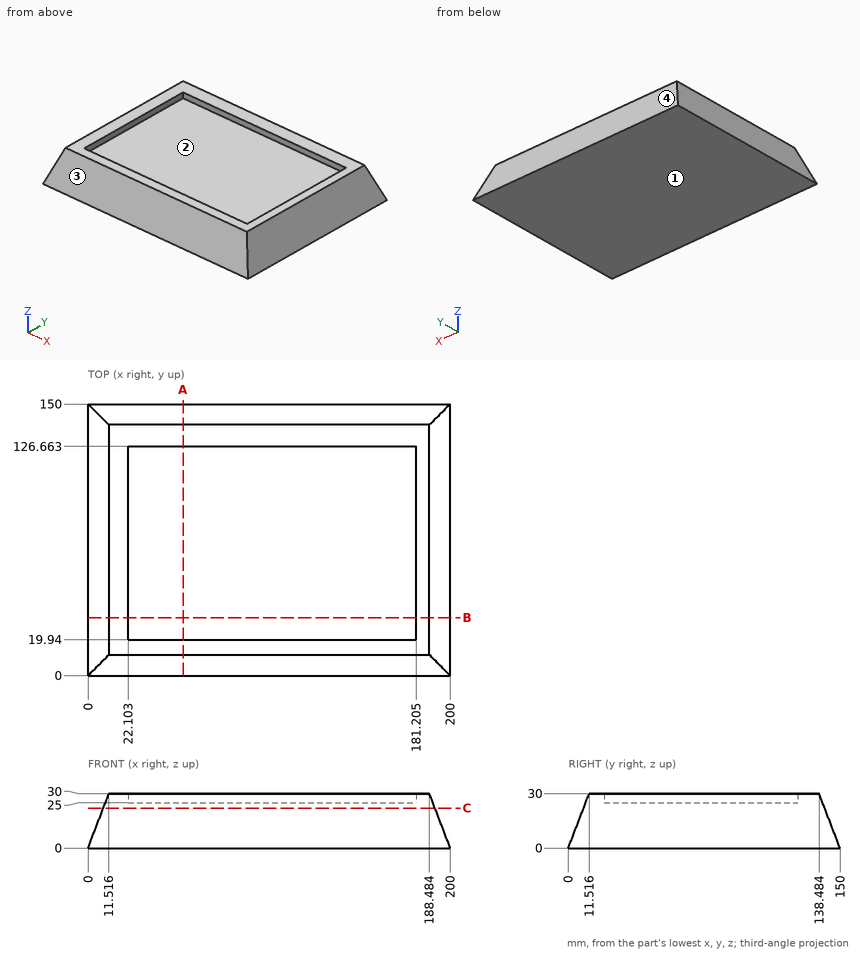
Could you check a few things on this drawing? It's one solid part, dimensions in mm from its lowest x, y, z. Give positions to 0.01 mm unless a question says otherwise; leave off trailing zeros. Order: outer loops, then holes, each group sorted by start corner. A loop starts at its lowest first (then second) coordinate and runs counter-clockwise, first axis right, second up. Notation, with made-up numbers: M 13,-35 L 23,-35 A22 cw 23,-28 Z; hole C -13.5,3 d6. An arc over 180 degrees is marked long. Use one line per item in the form item = value. Start each with the question number.
Item 1: If I drill on line 1 along Z through (x, y) = (99, 63); line 2 along X through (y, z) = (63, 26.5) (1 decimal); line 3 along Y through (x, z) = (94.5, 4) (1 decimal), over which ranges is the centre line in solid material (lowest first)?
Item 2: If we section it at C-C (z = 22): Write out the boundary of the cut face in (x, y) (1 decimal).
Item 3: If we section it at A-A (x = 52.5): Write out the boundary of the cut face in (y, z), then the cut area to 3 significant figures.
Item 4: We'd pull the mould along Y, two halves only. Please class the marked faces 1, 2, 3 and 4: +Y half, -Y half, draft (parallel to the pull), parting line (faces both ways), or undercut.
Item 5: Will these pins go through, and if not, where does the flat tip stop? pin 1 Ø12 at (x, y) = (41, 72.5) entering from +Z; pin 2 Ø5.5 at (y, z) = (48, 28) entering from +X; pin 3 Ø6 at (x, z) = (120.5, 8.5) entering from -Y.
Item 6: If we section it at B-B (y = 32): Write out the boundary of the cut face in (x, z) (1 decimal).
Outcome:
q1.line_1 = 0 to 25
q1.line_2 = 10.2 to 22.1, 181.2 to 189.8
q1.line_3 = 1.5 to 148.5
q2.outline = M 8.4,8.4 L 191.6,8.4 L 191.6,141.6 L 8.4,141.6 Z
q3.outline = M 0,0 L 150,0 L 138.48,30 L 126.66,30 L 126.66,25 L 19.94,25 L 19.94,30 L 11.52,30 Z
q3.area = 3,620 mm2
q4.face_1 = draft
q4.face_2 = undercut
q4.face_3 = -Y half
q4.face_4 = +Y half
q5.pin_1 = 25
q5.pin_2 = 190.31
q5.pin_3 = 2.11
q6.outline = M 0,0 L 200,0 L 188.5,30 L 181.2,30 L 181.2,25 L 22.1,25 L 22.1,30 L 11.5,30 Z
